```python
from build123d import *

# Parameters (mm, degrees)
BOSS_EXTRUDE1_DEPTH = 72
SKETCH2_R           = 4.25
CUT_EXTRUDE1_DEPTH  = 120.079805173
SKETCH3_R           = 6.35
BOSS_EXTRUDE2_DEPTH = 26
BOSS_EXTRUDE3_START = 26
SKETCH5_R           = 6.35
BOSS_EXTRUDE3_DEPTH = 26


with BuildPart() as part:
    # Sketch1 → Boss-Extrude1 (new body)
    with BuildSketch(Plane.XY):
        Polygon((-57.25, 32), (57.25, 32), (70, 32), (70, 26), (57.25, 26), (57.25, -32), (-57.25, -32), (-57.25, 26), (-70, 26), (-70, 32), align=None)
    extrude(amount=BOSS_EXTRUDE1_DEPTH)

    # Sketch2 → Cut-Extrude1 (cut, through all)
    with BuildSketch(Plane(origin=(0, 32, 0), x_dir=(1, 0, 0), z_dir=(0, 1, 0))):
        with Locations(Location((61.5, -36, 0), (0, 0, 180))):
            Circle(SKETCH2_R)
        with BuildLine():
            Line((-61.5, -31.5), (-70, -31.5))
            Line((-70, -31.5), (-70, -40.5))
            Line((-70, -40.5), (-61.5, -40.5))
            ThreePointArc((-61.5, -40.5), (-57, -36), (-61.5, -31.5))
        make_face()
    extrude(amount=-CUT_EXTRUDE1_DEPTH, mode=Mode.SUBTRACT)

    # Sketch3 → Boss-Extrude2 (add)
    with BuildSketch(Plane.XY.offset(72)):
        with Locations(Location((0, 0, 0), (0, 0, 180))):
            Circle(SKETCH3_R)
    extrude(amount=BOSS_EXTRUDE2_DEPTH)

    # Sketch5 → Boss-Extrude3 (add)
    with BuildSketch(Plane(origin=(0, 0, 0), x_dir=(-1, 0, 0), z_dir=(0, 0, -1)).offset(BOSS_EXTRUDE3_START)):
        Circle(SKETCH5_R)
    extrude(amount=-BOSS_EXTRUDE3_DEPTH)


solid = part.part
```
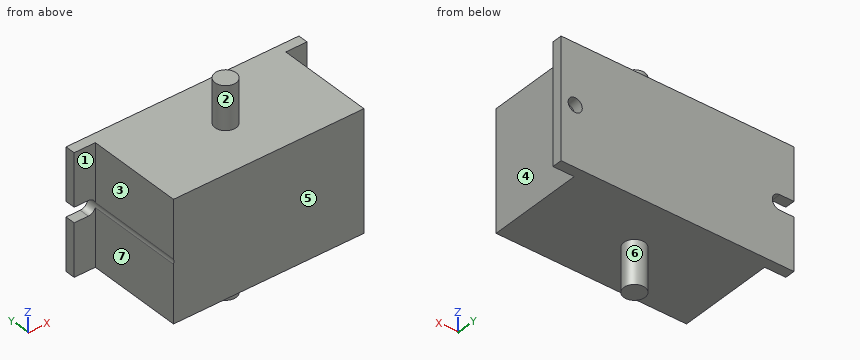
Source: CAD feature listing. Evaluate the final solid. Frame: model axes, mm. Face numbers are marked on the shaded views. A direction names the side the tool comes from. Coordinates: 2 decimals unless noted, no trailing zeros. Write each loop counter-clockwise with the first axis right and the second up, starting at its lowest first coordinate (ties: lowest second). Pieces come first, ordered by that corner, then holes. Notation, with made-up numbers: (75, 47) - (82, 47) arc R29 ccw to (82, 68) - close; hole circle Ø7 at (6.25, 83). An arc over 180 degrees is marked (long way). Answer as a JSON object with one key per item and string values.
Q1. Draft query along X for the marked faces 1, 2, 3 and 4. Return one class per face: released by +X, released by -X, zero draft, split by the parting line, or undercut.
Ans:
{"face 1": "zero draft", "face 2": "split by the parting line", "face 3": "released by -X", "face 4": "released by +X"}
Q2. Section query D-D, the plane y = -28. Output: boundary loops of the cut face in (x, z).
Ans:
{"outline": "(-57.25, 0) - (57.25, 0) - (57.25, 72) - (-57.25, 72) - (-57.25, 37.48) arc R4.5 cw to (-57.25, 34.52) - close"}
Q3. Material intervals for line 1 (Z direction, x = 61, y = 28); line 2 (Z direction, x = -53, y = 12); line 3 (X direction, y = -4, z = 63), sorted ascending. Write a range as [from, to].
Ans:
{"line 1": "z = [0, 31.78], [40.22, 72]", "line 2": "z = [0, 72]", "line 3": "x = [-57.25, 57.25]"}
Q4. Set-up query: the marked faces 5, 6 and 7. Return all of +Z, -Z, +X, -X, +Y, -Y with unobstructed straight access to the full face (end or side cutting, diameter ignored); none if empty.
Ans:
{"face 5": "+Z, -Z, +X, -X, -Y", "face 6": "-Z", "face 7": "+Z, -Z, -X, -Y"}
Q5. First-contact query: pin 1 Ø1.5 at (x, y) = (-36, -6.5) entering from +Z; pin 2 Ø10 at (x, z) = (-66.5, 18.5) entering from -Y; pin 3 Ø5 at (x, y) = (-66, 29) entering from -Z; pin 4 Ø19 at (x, y) = (-8.5, 12) entering from -Z. Flat tips, straight axial feed; report the tip coordinate or a pass-through.
Ans:
{"pin 1": "stops at z = 72", "pin 2": "stops at y = 26", "pin 3": "stops at z = 0", "pin 4": "stops at z = -26"}
Q6. Section query B-B, the plane y = 0. Output: boundary loops of the cut face in (x, z), plus the area to 3 significant figures.
Ans:
{"outline": "(-57.25, 0) - (-6.35, 0) - (-6.35, -26) - (6.35, -26) - (6.35, 0) - (57.25, 0) - (57.25, 72) - (6.35, 72) - (6.35, 98) - (-6.35, 98) - (-6.35, 72) - (-57.25, 72) - (-57.25, 37.48) arc R4.5 cw to (-57.25, 34.52) - close", "area": "8,900 mm2"}
Q7. Section query C-C, the plane z = 62.5. Output: boundary loops of the cut face in (x, y), plus the area to 3 significant figures.
Ans:
{"outline": "(-70, 26) - (-57.25, 26) - (-57.25, -32) - (57.25, -32) - (57.25, 26) - (70, 26) - (70, 32) - (-70, 32) - close", "area": "7,480 mm2"}
Q8. Section query A-A, the plane x = 0. Output: boundary loops of the cut face in (y, z), plus the area to 3 significant figures.
Ans:
{"outline": "(-32, 0) - (-6.35, 0) - (-6.35, -26) - (6.35, -26) - (6.35, 0) - (32, 0) - (32, 72) - (6.35, 72) - (6.35, 98) - (-6.35, 98) - (-6.35, 72) - (-32, 72) - close", "area": "5,270 mm2"}
